Model file for the job. Use its own axes, mm. A direction names the side the tool comes from. Give positions to 0.01 mm unless a question says otherwise; leave off trailing zeros. Loops run counter-clockwise (first coordinate to the right, second up) from the corner with the lowest first, then second, coordinate; pieces in that order, holes last. Notation, with made-up numbers: M 58.25,16 L 90.25,16 A11 cw 90.25,33 Z; hole C 73,19 d3. An arc over 180 degrees is marked long. Answer in a Markdown table with one row per item.
```python
from build123d import *

# Parameters (mm, degrees)
BOSS_EXTRUDE1_DEPTH = 4
SKETCH2_W           = 2.5
SKETCH2_H           = 4
CUT_EXTRUDE1_DEPTH  = 4


with BuildPart() as part:
    # Sketch1 → Boss-Extrude1 (new body)
    with BuildSketch(Plane.XY):
        with BuildLine():
            Line((0, 0), (10, 0))
            Line((10, 0), (10, 4))
            Line((10, 4), (12.5, 4))
            Line((12.5, 4), (12.5, 8))
            Line((12.5, 8), (10, 8))
            Line((10, 8), (10, 12))
            Line((10, 12), (14.8, 12))
            Line((14.8, 12), (14.8, 17))
            ThreePointArc((14.8, 17), (5, 26.8), (-4.8, 17))
            Line((-4.8, 17), (-4.8, 12))
            Line((-4.8, 12), (0, 12))
            Line((0, 12), (0, 8))
            Line((0, 8), (-2.5, 8))
            Line((-2.5, 8), (-2.5, 4))
            Line((-2.5, 4), (0, 4))
            Line((0, 4), (0, 0))
        make_face()
        Polygon((3.354551733, 18.071172359), (6.645448267, 18.071172359), (8.290896534, 20.921172359), (6.645448267, 23.771172359), (3.354551733, 23.771172359), (1.709103466, 20.921172359), align=None, mode=Mode.SUBTRACT)
        Polygon((8.290896534, 10.5), (6.645448267, 13.35), (3.354551733, 13.35), (1.709103466, 10.5), (3.354551733, 7.65), (6.645448267, 7.65), align=None, mode=Mode.SUBTRACT)
    extrude(amount=BOSS_EXTRUDE1_DEPTH)

    # Sketch2 → Cut-Extrude1 (cut)
    with BuildSketch(Plane.XY.offset(4)):
        with Locations((-1.25, 6)):
            Rectangle(SKETCH2_W, SKETCH2_H)
        with Locations((11.25, 6)):
            Rectangle(SKETCH2_W, SKETCH2_H)
    extrude(amount=-CUT_EXTRUDE1_DEPTH, mode=Mode.SUBTRACT)


solid = part.part
```
Q1. Saw through at A-A (x = 5). Give the cut face in (y, z).
Reported:
| item | result |
|---|---|
| outline | M 0,0 L 7.65,0 L 7.65,4 L 0,4 Z; M 13.35,0 L 18.07,0 L 18.07,4 L 13.35,4 Z; M 23.77,0 L 26.8,0 L 26.8,4 L 23.77,4 Z |
Q2. Saw through at C-C (y = 3.5). Give the cut face in (x, z).
Reported:
| item | result |
|---|---|
| outline | M 0,0 L 10,0 L 10,4 L 0,4 Z |
Q3. Probe probe 1 along Y at (x, z) = (6.25, 3.75); probe 2 along Y at (x, z) = (2.25, 1.2); probe 3 along X at (y, z) = (5.5, 2.95). List the from-to ranges inside material, lowest first.
Reported:
| item | result |
|---|---|
| probe 1 | 0 to 7.65, 13.35 to 18.07, 23.77 to 26.72 |
| probe 2 | 0 to 9.56, 11.44 to 19.98, 21.86 to 26.41 |
| probe 3 | 0 to 10 |
Q4. 3-axis set-ups, long thin cutter, end or side, ignore diameter. For faces 1 (the face through (2.52, 19.52, 1.97)), 2 (the face through (12, 12, 2)), 3 (the face through (-4.8, 15, 2)): which of +Z, -Z, +X, -X, +Y, -Y reach the whole face in a straight line?
Reported:
| item | result |
|---|---|
| face 1 | +Z, -Z |
| face 2 | +Z, -Z, +X, -Y |
| face 3 | +Z, -Z, -X, +Y, -Y |
Q5. Saw through at D-D (x = 2). Give the cut face in (y, z), and give its area (3 significant figures).
Reported:
| item | result |
|---|---|
| outline | M 0,0 L 10,0 L 10,4 L 0,4 Z; M 11,0 L 20.42,0 L 20.42,4 L 11,4 Z; M 21.43,0 L 26.33,0 L 26.33,4 L 21.43,4 Z |
| area | 97.3 mm² |
Q6. Drop flat-ended pins along their axis: pin 1 (1.2 mm diameter, centred on x = 12, z = 1.5, fed in from -Y); pin 2 (1.6 mm diameter, centred on x = 5, z = 1.5, fed in from -Y). Give the stop position or say it passes through.
Reported:
| item | result |
|---|---|
| pin 1 | y = 12 |
| pin 2 | y = 0 |
Q7. Mould opens along Y. For faces 4 (the face through (-2, 12, 2)), 5 (the face through (7.48, 11.905, 1.972)), 6 (the face through (5.215, 26.798, 1.972)) say: released by +Y, released by -Y, zero draft, split by the parting line, or undercut.
Reported:
| item | result |
|---|---|
| face 4 | released by -Y |
| face 5 | undercut |
| face 6 | released by +Y |
Q8. Saw through at B-B (z = 1.45). Give the cut face in (x, y), and give its area (3 significant figures).
Reported:
| item | result |
|---|---|
| outline | M -4.8,12 L 0,12 L 0,0 L 10,0 L 10,12 L 14.8,12 L 14.8,17 A9.8 ccw -4.8,17 Z; hole M 1.71,10.5 L 3.35,7.65 L 6.65,7.65 L 8.29,10.5 L 6.65,13.35 L 3.35,13.35 Z; hole M 1.71,20.92 L 3.35,18.07 L 6.65,18.07 L 8.29,20.92 L 6.65,23.77 L 3.35,23.77 Z |
| area | 313 mm² |
